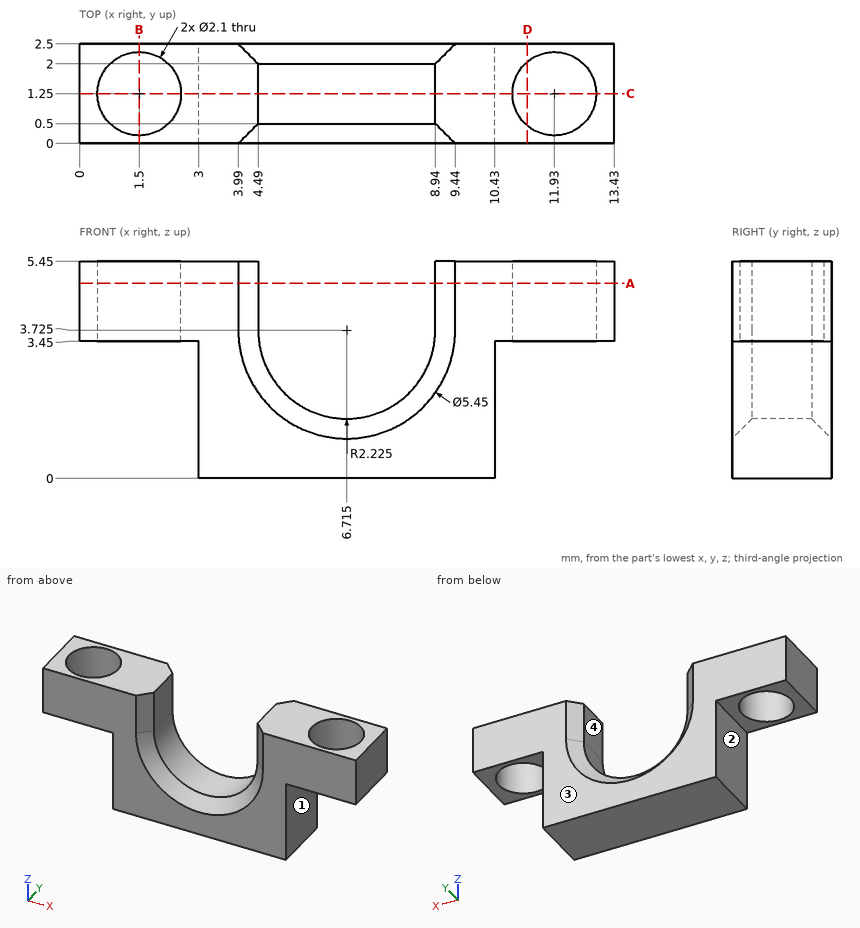
Answer from the drawing. Dimensions are ordinates in mm from the lowest x, y and z of the part. A direction names the side the tool comes from. Give positions to 0.01 mm unless a question says otherwise; leave off trailing zeros. Write each loop counter-clockwise with the first axis right and the second up, starting at its lowest first coordinate (ties: lowest second). Pieces come first, ordered by that corner, then holes.
1) Given P1, Ø1, axis at y = 1, z = 2, coming from the -X side; P2, Ø0.8, axis at x = 1, y = 0.5, coming from the -Z side; P3, Ø1, axis at x = 8.5, y = 1, coming from the +Z side; P4, Ø0.8, axis at y = 1, z = 2.5, coming from the +X side, each flat-ended and moving along its own axis, determine where each tip first touches the part or whether it passes through.
2) Section A-A (z = 4.9) is taken. Write down the section's boundary in (x, y), and give its area (3 significant figures).
3) Section C-C (y = 1.25) is taken. Count the separate pieces of the cut face and the enclosed holes in it.
4) Section B-B (x = 1.5) is taken. Write down the section's boundary in (y, z).
5) A tool of negligible diameter and unlimited length cuts with its end or side. For the marked faces 1, 2, 3 and 4, from which of +Z, -Z, +X, -X, +Y, -Y can it reach the whole face along a straight path? Write none if from no direction.
6) Section D-D (x = 11.25) is taken. Write down the section's boundary in (y, z).
7) Find the intervals of material crossed by L1, parallel to Y at x = 1.5, z = 4.95; L2, parallel to X at y = 1.55, z = 5.2 (1 decimal); L3, parallel to X at y = 2.15, z = 2.9, in increasing order.
Response:
1. P1: stops at x = 3
1. P2: stops at z = 3.45
1. P3: stops at z = 5.45
1. P4: stops at x = 10.43
2. outline: (0, 0) - (3.99, 0) - (4.49, 0.5) - (4.49, 2) - (3.99, 2.5) - (0, 2.5) - close; (8.94, 0.5) - (9.44, 0) - (13.43, 0) - (13.43, 2.5) - (9.44, 2.5) - (8.94, 2) - close; hole circle Ø2.1 at (1.5, 1.25); hole circle Ø2.1 at (11.93, 1.25)
2. area: 15.0 mm2
3. separate pieces: 3
3. enclosed holes: 0
4. outline: (0, 3.45) - (0.2, 3.45) - (0.2, 5.45) - (0, 5.45) - close; (2.3, 3.45) - (2.5, 3.45) - (2.5, 5.45) - (2.3, 5.45) - close
5. face 1: -Z, +X, +Y, -Y
5. face 2: -Z, -X, +Y, -Y
5. face 3: +Z, -Z, +X, -X, +Y
5. face 4: +Z, +Y, -Y
6. outline: (0, 3.45) - (0.45, 3.45) - (0.45, 5.45) - (0, 5.45) - close; (2.05, 3.45) - (2.5, 3.45) - (2.5, 5.45) - (2.05, 5.45) - close
7. L1: y = 0 to 0.2, 2.3 to 2.5
7. L2: x = 0 to 0.5, 2.5 to 4.5, 8.9 to 10.9, 12.9 to 13.4
7. L3: x = 3 to 4.49, 8.94 to 10.43
